Input: part model. Units: mm. Frame: model coordinates. A direction names the side the tool comes from. Coordinates: 2 decimals unless noted, no trailing zeros. Order: outer loops, then holes, each group sorted by start corner. A loop starts at its lowest first (then second) coordinate and runs counter-clockwise, first axis right, second up. Notation, with made-up numbers: (68, -34) -> (124, -34) arc R12 cw to (124, -19) -> close; hole circle Ø2 at (-11, 17.25). An arc over 180 degrees is marked (long way). One line per question, with ' | ' between items.
```python
from build123d import *

# Parameters (mm, degrees)
F0_W     = 76.2
F0_H     = 50.8
F0_R     = 3.5123065567
F0_R_2   = 12.7
F1_DEPTH = 12.7
F3_DEPTH = 2.54
F5_DEPTH = 50.8


with BuildPart() as f1:
    # F0 (on Top) → F1 (new body)
    with BuildSketch(Plane.XY):
        with Locations((-56.0851351521, 13.4954131208)):
            Rectangle(F0_W, F0_H)
        with Locations((-32.2128646076, 0)):
            Circle(F0_R, mode=Mode.SUBTRACT)
        with Locations((-54.8016801476, 15.0355538353)):
            Circle(F0_R_2, mode=Mode.SUBTRACT)
    extrude(amount=F1_DEPTH)

    # F2 (on face) → F3 (cut)
    with BuildSketch(Plane.XY.offset(12.7)):
        Polygon((-76.9599948415, 2.2896753244), (-80.2915843955, 4.5198883678), (-85.6237872068, 2.7123675299), (-85.8894135812, -1.2879801805), (-81.6579532121, -5.0020428543), (-78.0607372837, -3.2319081873), align=None)
        Polygon((-80.2915843955, 4.5198883678), (-85.281946506, 7.8605071594), (-85.6237872068, 2.7123675299), align=None)
        Polygon((-76.2417182173, 5.8927201535), (-80.2915843955, 4.5198883678), (-76.9599948415, 2.2896753244), align=None)
        Polygon((-72.6724954905, -0.5804372213), (-76.9599948415, 2.2896753244), (-78.0607372837, -3.2319081873), align=None)
        Polygon((-78.8967631712, -7.4256110723), (-78.0607372837, -3.2319081873), (-81.6579532121, -5.0020428543), align=None)
        Polygon((-81.6579532121, -5.0020428543), (-85.8894135812, -1.2879801805), (-86.2872932638, -7.2800699381), align=None)
        Polygon((-85.8894135812, -1.2879801805), (-85.6237872068, 2.7123675299), (-89.1032538719, 1.5328909188), align=None)
        Polygon((-84.5270859868, 32.4696852051), (-86.0750453988, 31.0185304322), (-86.9942569946, 29.1061814688), (-87.1605761549, 26.990911639), (-86.5515405552, 24.9583998544), (-85.2494038283, 23.2831480942), (-83.4300267543, 22.1914083914), (-81.3391262888, 21.8306262424), (-79.2590901256, 22.2495272756), (-77.4708386744, 23.3915365852), (-76.2158852028, 25.102419486), (-75.6637181311, 27.1511117617), (-75.8889106819, 29.2609261685), (-76.8610493535, 31.1469205797), (-78.4488414314, 32.5543809995), (-80.4378467972, 33.2932220992), (-82.5594392549, 33.2636592941), align=None)
    extrude(amount=-F3_DEPTH, mode=Mode.SUBTRACT)

    # F4 (on face) → F5 (cut)
    with BuildSketch(Plane.XZ.offset(11.9045868792)):
        Polygon((-26.6611795004, 1.1490697949), (-22.6668310289, 9.9366341741), (-32.2742592543, 9.0020592324), align=None)
        Polygon((-85.6983154144, 1.6102975211), (-81.7039669428, 10.3978619002), (-91.3113951683, 9.4632869586), align=None)
    extrude(amount=-F5_DEPTH, mode=Mode.SUBTRACT)


solid = f1.part
```
1. Cut plane B-B, the plane y = 12.5. Return loops of the section in (x, z).
Recorded:
outline: (-94.19, 0) -> (-67.25, 0) -> (-67.25, 12.7) -> (-94.19, 12.7) -> close; (-42.36, 0) -> (-17.99, 0) -> (-17.99, 12.7) -> (-42.36, 12.7) -> close; hole (-91.31, 9.46) -> (-85.7, 1.61) -> (-81.7, 10.4) -> close; hole (-32.27, 9) -> (-26.66, 1.15) -> (-22.67, 9.94) -> close
2. Cut plane D-D, the plane y = 26. Return loops of the section in (x, z), and give its area (3 significant figures).
Recorded:
outline: (-94.19, 0) -> (-61.21, 0) -> (-61.21, 12.7) -> (-75.97, 12.7) -> (-75.97, 10.16) -> (-81.81, 10.16) -> (-85.7, 1.61) -> (-91.31, 9.46) -> (-84.15, 10.16) -> (-86.86, 10.16) -> (-86.86, 12.7) -> (-94.19, 12.7) -> close; (-48.39, 0) -> (-17.99, 0) -> (-17.99, 12.7) -> (-48.39, 12.7) -> close; hole (-32.27, 9) -> (-26.66, 1.15) -> (-22.67, 9.94) -> close | area: 697 mm^2
3. Pin query (flat end, axial travel): pin 1 Ø0.9 at (x, y) = (-85, 27) entering from +Z. Return the tip coordinate at first contact, or that it passes through.
Recorded:
pin 1: stops at z = 10.16
4. Ray query, line 1 (X direction, y = -2, z = 2.5); line 2 (X direction, y = 6.5, z = 6); line 3 (X direction, y = 25, z = 12). Return the intervals inside material, ascending. Write a range as [from, to].
Recorded:
line 1: x = [-94.19, -86.33], [-85.29, -35.1], [-29.33, -27.63], [-26.05, -17.99] | line 2: x = [-94.19, -88.84], [-83.7, -64.21], [-45.4, -30.13], [-24.46, -17.99] | line 3: x = [-94.19, -86.56], [-76.29, -62.68], [-46.93, -17.99]
5. Cut plane A-A, the plane z = 6.75. Return loops of the section in (x, y), and give its area (3 significant figures).
Recorded:
outline: (-94.19, -11.9) -> (-89.37, -11.9) -> (-89.37, 38.9) -> (-94.19, 38.9) -> close; (-83.36, -11.9) -> (-30.66, -11.9) -> (-30.66, -3.15) arc R3.51 cw (long way) to (-30.66, 3.15) -> (-30.66, 38.9) -> (-83.36, 38.9) -> close; (-24.12, -11.9) -> (-17.99, -11.9) -> (-17.99, 38.9) -> (-24.12, 38.9) -> close; hole circle Ø25.4 at (-54.8, 15.04) | area: 2,700 mm^2
6. Access query for faces 1 (the face through (-84.352, 22.745, 11.448)), 2 (the face through (-65, 25, 0)). Directions: +Z, -Z, +X, -X, +Y, -Y. A direction counts if a zero-diameter tool reaches every point of the face in a straight line with its end or side. Return the directions, or none.
Recorded:
face 1: +Z | face 2: -Z, +X, -X, +Y, -Y
7. Cut plane C-C, the plane x = -58. Return loops of the section in (y, z).
Recorded:
outline: (-11.9, 0) -> (2.74, 0) -> (2.74, 12.7) -> (-11.9, 12.7) -> close; (27.33, 0) -> (38.9, 0) -> (38.9, 12.7) -> (27.33, 12.7) -> close
8. Mould query, pull axis Y, two halves, no side actions, for faces 3 (the face through (-86, 28, 10.16)), 4 (the face through (-57, 38.895, 6)), 5 (the face through (-79, 28, 10.16)), 6 (the face through (-94.185, 13, 6)). Classes: released by +Y, released by -Y, zero draft, split by the parting line, or undercut.
Recorded:
face 3: undercut | face 4: released by +Y | face 5: undercut | face 6: zero draft
